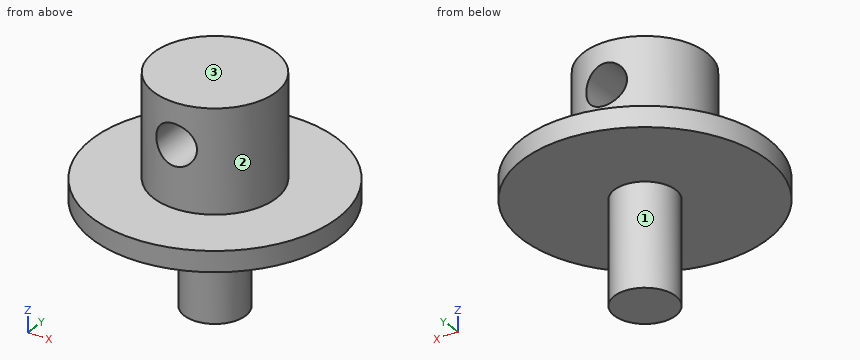
from build123d import *

# Parameters (mm, degrees)
ESQUISSE1_R                  = 1.5
BOSS_EXTRU_1_DEPTH           = 5
ESQUISSE2_R                  = 6
BOSS_EXTRU_2_DEPTH           = 1
ESQUISSE3_R                  = 3
BOSS_EXTRU_3_DEPTH           = 5
ESQUISSE4_R                  = 1
ENL_V_MAT_EXTRU_1_DEPTH      = 5
ENL_V_MAT_EXTRU_1_DEPTH_BACK = 5


with BuildPart() as part:
    # Esquisse1 → Boss.-Extru.1 (new body)
    with BuildSketch(Plane.XY):
        Circle(ESQUISSE1_R)
    extrude(amount=BOSS_EXTRU_1_DEPTH)

    # Esquisse2 → Boss.-Extru.2 (add)
    with BuildSketch(Plane.XY.offset(5)):
        Circle(ESQUISSE2_R)
    extrude(amount=BOSS_EXTRU_2_DEPTH)

    # Esquisse3 → Boss.-Extru.3 (add)
    with BuildSketch(Plane.XY.offset(6)):
        Circle(ESQUISSE3_R)
    extrude(amount=BOSS_EXTRU_3_DEPTH)

    # Esquisse4 → Enl_v. mat.-Extru.1 (cut, two sides)
    with BuildSketch(Plane(origin=(0, 0, 0), x_dir=(1, 0, 0), z_dir=(0, 1, 0))) as enl_v_mat_extru_1_sk:
        with Locations((0, -9)):
            Circle(ESQUISSE4_R)
    extrude(amount=ENL_V_MAT_EXTRU_1_DEPTH, mode=Mode.SUBTRACT)
    extrude(enl_v_mat_extru_1_sk.sketch, amount=-ENL_V_MAT_EXTRU_1_DEPTH_BACK, mode=Mode.SUBTRACT)


solid = part.part
Model file for the job. Use its own axes, mm. Face numbers are marked on the shaded views. A direction names the side the tool comes from. Give positions to 0.01 mm unless a question says otherwise; leave off trailing zeros. Write each loop counter-clockwise with the first axis right and the second up, starting at its lowest first coordinate (ties: lowest second). Pieces come first, ordered by that corner, then holes. Notation, with made-up numbers: M 54.5,30.5 L 112.5,30.5 A24 ccw 112.5,57.5 Z; hole C 13,11 d5. An arc over 180 degrees is marked long. One line per item, written item: value. Start each with the question number.
Q1. Drop flat-ended pins along their axis: pin 1 Ø1.5 at (x, z) = (-2, 2.5) entering from +Y; pin 2 Ø1.2 at (x, z) = (0, 9) entering from -Y; pin 3 Ø2 at (x, z) = (-1.5, 9) entering from -Y; pin 4 Ø4 at (y, z) = (-1, 2.5) entering from -X. Give the stop position or say it passes through.
Q2. Saw through at A-A, the plane x = 0. Write the cut outline in (y, z), plus the area to 3 significant figures.
Q3. Saw through at B-B, the plane x = -2.5. Write the cut outline in (y, z).
Q4. 3-axis set-ups, long thin cutter, end or side, ignore diameter. For the marked faces 1, 2 and 3: which of +Z, -Z, +X, -X, +Y, -Y reach the whole face in a straight line?
Q5. Probe probe 1 along Z at (x, y) = (0, 1.15); probe 2 along Z at (x, y) = (0, -1.9); probe 3 along Z at (x, y) = (2.75, 2.5). List the from-to ranges inside material, lowest first. Write a range as [from, to].
Q6. Saw through at D-D, the plane z = 4.5. Write the cut outline in (x, y).
Q7. Saw through at C-C, the plane z = 8.75. Write the cut outline in (x, y).
Output values:
1. pin 1: stops at y = 0.83
1. pin 2: passes through
1. pin 3: stops at y = -2.9
1. pin 4: stops at x = -1.5
2. outline: M -6,5 L -1.5,5 L -1.5,0 L 1.5,0 L 1.5,5 L 6,5 L 6,6 L 3,6 L 3,8 L -3,8 L -3,6 L -6,6 Z; M -3,10 L 3,10 L 3,11 L -3,11 Z
2. area: 45.0 mm²
3. outline: M -5.45,5 L 5.45,5 L 5.45,6 L 1.66,6 L 1.66,11 L -1.66,11 L -1.66,6 L -5.45,6 Z
4. face 1: -Z
4. face 2: +Z
4. face 3: +Z, +X, -X, +Y, -Y
5. probe 1: z = [0, 8], [10, 11]
5. probe 2: z = [5, 8], [10, 11]
5. probe 3: z = [5, 6]
6. outline: C 0,0 d3
7. outline: M -0.97,-2.84 L -0.97,2.84 A3 ccw Z; M 0.97,-2.84 A3 ccw 0.97,2.84 Z
